The model under review builds one solid part; all positions refer to its coordinate system, in mm. Face numbers are marked on the shaded views. A direction names the side the tool comes from. Round coordinates to 2 decimals unless told otherwise and drop trailing zeros. Write each loop counter-clockwise with the first axis right and the second up, starting at its lowest first coordinate (ties: lowest second). Pieces come first, ordered by that corner, then holes. Notation, with made-up numbers: (87, 19) -> (120, 19) arc R10 cw to (120, 30) -> close; hole circle Ø7 at (11, -23). An arc over 180 degrees is marked (long way). Use CSV: the item, a comma, the result in double quotes. Start each with the question number.
1) Take a section at B-B, the plane z = 12. State how many separate pieces and enclosed holes the cut face has, then the cut area to 3 significant figures.
2) Take a section at C-C, the plane x = -55. Give the boundary of the cut face in (y, z), then the cut area to 3 significant figures.
3) Take a section at D-D, the plane z = -33. Give the boundary of the cut face in (x, y).
4) Take a section at A-A, the plane y = -8. Give the boundary of the cut face in (x, z), then the cut area to 3 significant figures.
5) Mouldability with a two-part tool opening along X and no side actions: class the marked faces 6, 7 and 8 as released by +X, released by -X, zero draft, split by the parting line, or undercut.
6) Machinability: for the marked faces 1, 2, 3, 4 and 5, which of the approach directions +Z, -Z, +X, -X, +Y, -Y give a long, thin tool a straight path to every point of the face, cutting with its end or side? Answer none if there is none.
7) For pin 1 Ø9.5 at (y, z) = (42, -65) entering from +X; pin 2 Ø6 at (y, z) = (-8, 23) entering from -X; pin 3 Ø5 at (x, z) = (-61, -5.5) entering from +Y, all flat-tipped, find the tip position at first contact; note any pin that passes through.
8) Wall thickness on probe 1 along X at (y, z) = (-20.25, 12); probe 2 along X at (y, z) = (-9.5, 13); probe 3 along Z at (x, y) = (55, -20.75): over which ranges is each line inside the solid? List them lowest first. Write a range as [from, to].
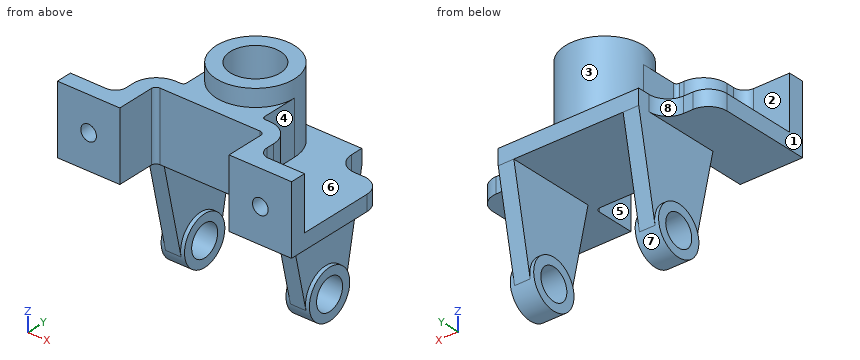
from build123d import *

# Parameters (mm, degrees)
BOSS_EXTRUDE2_DEPTH  = 10
SKETCH2_R            = 25
SKETCH2_R_2          = 16
BOSS_EXTRUDE4_DEPTH  = 45
BOSS_EXTRUDE5_START  = 34
BOSS_EXTRUDE5_DEPTH  = 34
SKETCH4_R            = 5
CUT_EXTRUDE1_DEPTH   = 34
SKETCH6_R            = 15.5
SKETCH6_R_2          = 10
BOSS_EXTRUDE6_DEPTH  = 7.5
BOSS_EXTRUDE8_DEPTH  = 5
SKETCH8_R            = 15.5
SKETCH8_R_2          = 10
BOSS_EXTRUDE9_DEPTH  = 7.5
BOSS_EXTRUDE10_DEPTH = 5


with BuildPart() as part:
    # Sketch1 → Boss-Extrude2 (new body)
    with BuildSketch(Plane.XY):
        with BuildLine():
            Line((-32, 0), (32, 0))
            ThreePointArc((32, 0), (34.121320344, -0.878679656), (35, -3))
            Line((35, -3), (35, -27.235915493))
            Line((35, -27.235915493), (75, -27.235915493))
            Line((75, -27.235915493), (75, 30.764084507))
            ThreePointArc((75, 30.764084507), (71.485281374, 39.249365881), (63, 42.764084507))
            Line((63, 42.764084507), (57, 42.764084507))
            ThreePointArc((57, 42.764084507), (48.514718626, 46.278803133), (45, 54.764084507))
            Line((45, 54.764084507), (45, 62.764084507))
            Line((45, 62.764084507), (-45, 62.764084507))
            Line((-45, 62.764084507), (-45, 54.764084507))
            ThreePointArc((-45, 54.764084507), (-48.514718626, 46.278803133), (-57, 42.764084507))
            Line((-57, 42.764084507), (-63, 42.764084507))
            ThreePointArc((-63, 42.764084507), (-71.485281374, 39.249365881), (-75, 30.764084507))
            Line((-75, 30.764084507), (-75, -27.235915493))
            Line((-75, -27.235915493), (-35, -27.235915493))
            Line((-35, -27.235915493), (-35, -3))
            ThreePointArc((-35, -3), (-34.121320344, -0.878679656), (-32, 0))
        make_face()
    extrude(amount=-BOSS_EXTRUDE2_DEPTH)

    # Sketch2 → Boss-Extrude4 (add)
    with BuildSketch(Plane.XY):
        with Locations(Location((0, 35, 0), (0, 0, 180))):
            Circle(SKETCH2_R)
        with Locations(Location((0, 35, 0), (0, 0, 180))):
            Circle(SKETCH2_R_2, mode=Mode.SUBTRACT)
    extrude(amount=BOSS_EXTRUDE4_DEPTH)

    # Sketch3 → Boss-Extrude5 (add)
    with BuildSketch(Plane.XY.offset(BOSS_EXTRUDE5_START)):
        with BuildLine():
            Line((-75, -17.235915493), (-52, -17.235915493))
            ThreePointArc((-52, -17.235915493), (-47.050252532, -15.185662961), (-45, -10.235915493))
            Line((-45, -10.235915493), (-45, -5))
            ThreePointArc((-45, -5), (-40.606601718, 5.606601718), (-30, 10))
            Line((-30, 10), (-27, 10))
            ThreePointArc((-27, 10), (-25.585786438, 10.585786438), (-25, 12))
            Line((-25, 12), (-25, 35))
            ThreePointArc((-25, 35), (0, 10), (25, 35))
            Line((25, 35), (25, 12))
            ThreePointArc((25, 12), (25.585786438, 10.585786438), (27, 10))
            Line((27, 10), (30, 10))
            ThreePointArc((30, 10), (40.606601718, 5.606601718), (45, -5))
            Line((45, -5), (45, -10.235915493))
            ThreePointArc((45, -10.235915493), (47.050252532, -15.185662961), (52, -17.235915493))
            Line((52, -17.235915493), (75, -17.235915493))
            Line((75, -17.235915493), (75, -27.235915493))
            Line((75, -27.235915493), (35, -27.235915493))
            Line((35, -27.235915493), (35, -3))
            ThreePointArc((35, -3), (34.121320344, -0.878679656), (32, 0))
            Line((32, 0), (-32, 0))
            ThreePointArc((-32, 0), (-34.121320344, -0.878679656), (-35, -3))
            Line((-35, -3), (-35, -27.235915493))
            Line((-35, -27.235915493), (-75, -27.235915493))
            Line((-75, -27.235915493), (-75, -17.235915493))
        make_face()
    extrude(amount=-BOSS_EXTRUDE5_DEPTH)

    # Sketch4 → Cut-Extrude1 (cut)
    with BuildSketch(Plane.XZ.offset(27.235915493)):
        with Locations(Location((-55, 12, 0), (0, 0, 270))):
            Circle(SKETCH4_R)
        with Locations(Location((55, 12, 0), (0, 0, 270))):
            Circle(SKETCH4_R)
    extrude(amount=-CUT_EXTRUDE1_DEPTH, mode=Mode.SUBTRACT)



with BuildPart() as body_2:
    # Sketch6 → Boss-Extrude6 (new, symmetric)
    with BuildSketch(Plane(origin=(40, 0, 0), x_dir=(0, 0, -1), z_dir=(1, 0, 0))):
        with Locations((70, 35)):
            Circle(SKETCH6_R)
        with Locations((70, 35)):
            Circle(SKETCH6_R_2, mode=Mode.SUBTRACT)
    extrude(amount=BOSS_EXTRUDE6_DEPTH, both=True)


with BuildPart() as part_1:
    add(part.part)

    add(body_2.part)  # Boss-Extrude8 merges body 2
    # Sketch7 → Boss-Extrude8 (add, symmetric)
    with BuildSketch(Plane(origin=(40, 0, 0), x_dir=(0, 0, -1), z_dir=(1, 0, 0))):
        with BuildLine():
            Line((10, 62.764084507), (73.029857486, 50.200985613))
            ThreePointArc((73.029857486, 50.200985613), (54.50102976, 34.821334149), (73.379467389, 19.872898488))
            Line((73.379467389, 19.872898488), (10, 5.71361999))
            Line((10, 5.71361999), (10, 62.764084507))
        make_face()
    extrude(amount=BOSS_EXTRUDE8_DEPTH, both=True)



with BuildPart() as body_2_2:
    # Sketch8 → Boss-Extrude9 (new, symmetric)
    with BuildSketch(Plane(origin=(-40, 0, 0), x_dir=(0, 0, -1), z_dir=(1, 0, 0))):
        with Locations((70, 35)):
            Circle(SKETCH8_R)
        with Locations((70, 35)):
            Circle(SKETCH8_R_2, mode=Mode.SUBTRACT)
    extrude(amount=BOSS_EXTRUDE9_DEPTH, both=True)


with BuildPart() as part_2:
    add(part_1.part)

    add(body_2_2.part)  # Boss-Extrude10 merges body 2 2
    # Sketch9 → Boss-Extrude10 (add, symmetric)
    with BuildSketch(Plane(origin=(-40, 0, 0), x_dir=(0, 0, -1), z_dir=(1, 0, 0))):
        with BuildLine():
            Line((73.029857486, 50.200985613), (10, 62.764084507))
            Line((10, 62.764084507), (10, 5.71361999))
            Line((10, 5.71361999), (73.379467389, 19.872898488))
            ThreePointArc((73.379467389, 19.872898488), (54.50102976, 34.821334149), (73.029857486, 50.200985613))
        make_face()
    extrude(amount=BOSS_EXTRUDE10_DEPTH, both=True)


solid = part_2.part
Values found:
1,separate pieces,"3"
1,enclosed holes,"1"
1,area,"3,200 mm²"
2,outline,"(-27.24, -10) -> (42.93, -10) -> (42.93, 0) -> (-17.24, 0) -> (-17.24, 7) -> (-27.24, 7) -> close; (-27.24, 17) -> (-17.24, 17) -> (-17.24, 34) -> (-27.24, 34) -> close"
2,area,"942 mm²"
3,outline,"(-45, 10.85) -> (-35, 10.85) -> (-35, 58.18) -> (-45, 58.18) -> close; (35, 10.85) -> (45, 10.85) -> (45, 58.18) -> (35, 58.18) -> close"
4,outline,"(-75, -10) -> (-35, -10) -> (-35, 34) -> (-45, 34) -> (-45, 0) -> (-75, 0) -> close; (35, -10) -> (75, -10) -> (75, 0) -> (45, 0) -> (45, 34) -> (35, 34) -> close"
4,area,"1,480 mm²"
5,face 6,"zero draft"
5,face 7,"undercut"
5,face 8,"released by -X"
6,face 1,"+Z, -Z, -X, +Y, -Y"
6,face 2,"+Z, -X, +Y"
6,face 3,"+Z"
6,face 4,"+Z, +X, +Y"
6,face 5,"+Z, -Z, -Y"
7,pin 1,"x = 47.5"
7,pin 2,"x = -45.04"
7,pin 3,"y = 42.76"
8,probe 1,"[-75, -60], [-50, -35], [35, 50], [60, 75]"
8,probe 2,"[-45, -35], [35, 45]"
8,probe 3,"[-10, 7], [17, 34]"
